Could you check a few things on this model? Use its own coordinates, in mm. Face numbers are marked on the shaded views. A direction names the side the tool comes from. Give positions to 0.01 mm unless a question says otherwise; leave off trailing zeros. Write each loop counter-clockwise with the first axis right and the second up, starting at its lowest first coordinate (ties: lowest second). Pieces come first, ordered by that corner, then holes. Notation, with made-up numbers: M -26.5,56 L -7.5,56 A22 ccw -7.5,78 Z; hole C 35,81 d6. An arc over 180 degrees is marked long. Answer as a JSON object with one key per item and string values. Group by question number.
```python
from build123d import *

# Parameters (mm, degrees)
SKETCH1_R           = 31.5
BOSS_EXTRUDE1_DEPTH = 42
SKETCH2_R           = 31.5
BOSS_EXTRUDE2_DEPTH = 6
CHAMFER1_SIZE       = 6
SKETCH4_R           = 31.5
BOSS_EXTRUDE3_DEPTH = 8
CHAMFER2_SIZE       = 8
SKETCH6_R           = 7.5
BOSS_EXTRUDE4_DEPTH = 1
SKETCH7_R           = 4
BOSS_EXTRUDE5_DEPTH = 24
SKETCH10_R          = 2
CUT_EXTRUDE4_DEPTH  = 8
CUT_EXTRUDE5_DEPTH  = 10


with BuildPart() as part:
    # Sketch1 → Boss-Extrude1 (new body)
    with BuildSketch(Plane.XY):
        with Locations(Location((0, 0, 0), (0, 0, 180))):
            Circle(SKETCH1_R)
    extrude(amount=BOSS_EXTRUDE1_DEPTH)

    # Sketch2 → Boss-Extrude2 (add)
    with BuildSketch(Plane.XY.offset(42)):
        with Locations(Location((0, 0, 0), (0, 0, 180))):
            Circle(SKETCH2_R)
    extrude(amount=BOSS_EXTRUDE2_DEPTH)

    # Chamfer1
    chamfer1_edges = [part.edges().sort_by_distance(p)[0] for p in [
        (31.5, 0, 48),
    ]]
    chamfer(chamfer1_edges, length=CHAMFER1_SIZE)

    # Sketch4 → Boss-Extrude3 (add)
    with BuildSketch(Plane(origin=(0, 0, 0), x_dir=(-1, 0, 0), z_dir=(0, 0, -1))):
        Circle(SKETCH4_R)
    extrude(amount=BOSS_EXTRUDE3_DEPTH)

    # Chamfer2
    chamfer2_edges = [part.edges().sort_by_distance(p)[0] for p in [
        (31.5, 0, -8),
    ]]
    chamfer(chamfer2_edges, length=CHAMFER2_SIZE)

    # Sketch6 → Boss-Extrude4 (add)
    with BuildSketch(Plane(origin=(0, 0, -8), x_dir=(-1, 0, 0), z_dir=(0, 0, -1))):
        Circle(SKETCH6_R)
    extrude(amount=BOSS_EXTRUDE4_DEPTH)

    # Sketch7 → Boss-Extrude5 (add)
    with BuildSketch(Plane.XY.offset(48)):
        Circle(SKETCH7_R)
    extrude(amount=BOSS_EXTRUDE5_DEPTH)

    # Sketch10 → Cut-Extrude4 (cut)
    with BuildSketch(Plane.XY.offset(48)):
        with Locations((0, 15.2)):
            Circle(SKETCH10_R)
        with Locations((0, 22.2)):
            Circle(SKETCH10_R)
        with Locations((22.2, 0)):
            Circle(SKETCH10_R)
        with Locations((15.2, 0)):
            Circle(SKETCH10_R)
        with Locations((0, -22.2)):
            Circle(SKETCH10_R)
        with Locations((0, -15.2)):
            Circle(SKETCH10_R)
        with Locations((-22.2, 0)):
            Circle(SKETCH10_R)
        with Locations((-15.2, 0)):
            Circle(SKETCH10_R)
    extrude(amount=-CUT_EXTRUDE4_DEPTH, mode=Mode.SUBTRACT)

    # Sketch11 → Cut-Extrude5 (cut)
    with BuildSketch(Plane(origin=(2.5, 0, 0), x_dir=(0, 0, -1), z_dir=(1, 0, 0))):
        with BuildLine():
            Line((-67.418537693, 1.5), (-53.527084748, 1.5))
            ThreePointArc((-53.527084748, 1.5), (-52.027084748, 0), (-53.527084748, -1.5))
            Line((-53.527084748, -1.5), (-67.418537693, -1.5))
            ThreePointArc((-67.418537693, -1.5), (-68.918537693, 0), (-67.418537693, 1.5))
        make_face()
    extrude(amount=CUT_EXTRUDE5_DEPTH, mode=Mode.SUBTRACT)


solid = part.part
```
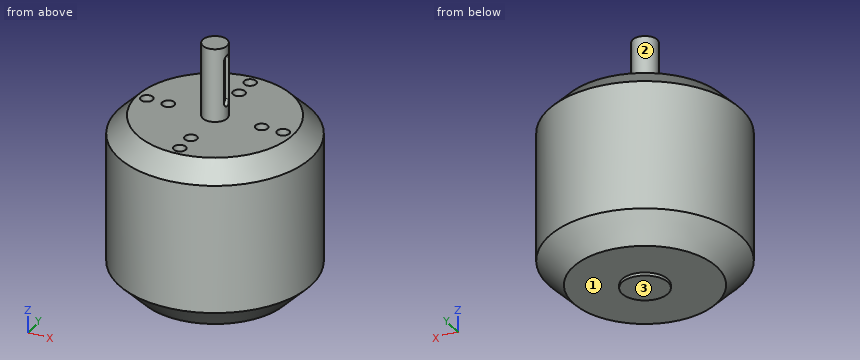
1) If we section it at B-B, the plane z = 58: List the corners of the cut face in (x, y) for me, plus the area to 3 significant figures.
2) Please list where these lines run through material, in increasing order: line 1 along Y through (x, z) = (0, 42.5); line 2 along Z through (x, y) = (-21, -8); line 3 along Y through (x, z) = (0, 45). Write a range as from..to.
3) I'm going to push flat-ended pins straight in: pin 1 (1.5 mm diameter, centred on x = -11.5, y = -23, fed in from -Z); pin 2 (5 mm diameter, centred on x = -17, z = 8, fed in from +Y); pin 3 (2 mm diameter, centred on x = 0.5, y = 23, fed in from +Z). Where does each tip first touch, or does it pass through?
4) If we section it at A-A, the plane z = 46.5: Give the number of separate pieces and of enclosed holes in the cut face, plus the area to 3 significant figures.
5) If we section it at D-D, the plane z = -4: List the corners of the cut face in (x, y) for me.
6) If we section it at C-C, the plane z = 4.5: List the corners of the cut face in (x, y) for me.
7) For the marked faces 1, 2 and 3, which set-ups out of +Z, -Z, +X, -X, +Y, -Y let a thin tool reach every point of the face, with its end or its side?
Taken from the geometry:
{
 "1": {"outline": "M 2.5,-1.5 L 2.5,1.5 L 3.71,1.5 A4 ccw long 3.71,-1.5 Z", "area": "46.1 mm²"},
 "2": {"line 1": "-31..-24.2, -20.2..-17.2, -13.2..13.2, 17.2..20.2, 24.2..31", "line 2": "-8..48", "line 3": "-28.5..-24.2, -20.2..-17.2, -13.2..13.2, 17.2..20.2, 24.2..28.5"},
 "3": {"pin 1": "z = -6.54", "pin 2": "y = 27.96", "pin 3": "z = 40"},
 "4": {"separate pieces": "1", "enclosed holes": "8", "area": "2,190 mm²"},
 "5": {"outline": "C 0,0 d55"},
 "6": {"outline": "C 0,0 d63"},
 "7": {"face 1": "-Z", "face 2": "+Z", "face 3": "-Z, +X, -X, +Y, -Y"}
}
